Design review of the part built by this model. Coordinates are the model's own, in mm. A direction names the side the tool comes from. Give positions to 0.01 mm unless a question says otherwise; leave off trailing zeros. Write each loop counter-clockwise with the first axis right and the second up, starting at its lowest first coordinate (ties: lowest second). Pieces come first, ordered by that corner, then holes. Notation, with made-up numbers: M 39,78 L 61,78 A10 ccw 61,87 Z; hole C -28,6.25 d3. An arc over 180 degrees is marked long. Answer in a Markdown table with one row per item.
Autodesk Fusion 360 part; units mm, degrees
sketch "Sketch1" plane through (0, 0, 0) normal (0, 1, 0) x (1, 0, 0)
  line L0 (15, 32.5) -> (-15, 32.5)
  line L1 (-15, 32.5) -> (-15, -32.5)
  line L2 (-15, -32.5) -> (15, -32.5)
  line L3 (15, -32.5) -> (15, 32.5)
  line L4 (15, 32.5) -> (-15, -32.5) construction
  line L5 (-15, 32.5) -> (15, -32.5) construction
  dimension "d1" = 30
  dimension "d2" = 65
extrude "Extrude1" add sketch "Sketch1" along normal blind 2
sketch "Sketch2" plane through (0, 2, 0) normal (0, 1, 0) x (-1, 0, 0)
  line L0 (-15, 32.5) -> (-15, -32.5)
  line L1 (-15, -32.5) -> (15, -32.5)
  line L2 (15, -32.5) -> (15, 32.5)
  line L3 (15, 32.5) -> (-15, 32.5)
  circle A0 centre (-11.5, -29) radius 2.8
  circle A1 centre (11.5, -29) radius 2.8
  circle A2 centre (-11.5, 29) radius 2.8
  circle A3 centre (11.5, 29) radius 2.8
  dimension "d5" = 5.6
  dimension "d6" = 3.5
  dimension "d7" = 3.5
  dimension "d8" = 5.6
  dimension "d9" = 3.5
  dimension "d10" = 3.5
  dimension "d11" = 5.6
  dimension "d12" = 3.5
  dimension "d13" = 3.5
  dimension "d14" = 5.6
  dimension "d15" = 3.5
  dimension "d16" = 3.5
extrude "Extrude2" add sketch "Sketch2" along normal blind 21 contours A0 | A1 | A2 | A3
sketch "Sketch3" plane through (0, 23, 0) normal (0, 1, 0) x (-1, 0, 0)
  circle A0 centre (-11.5, -29) radius 2.8
  circle A1 centre (-11.5, -29) radius 1.2
  circle A2 centre (11.5, -29) radius 1.2
  circle A3 centre (11.5, -29) radius 2.8
  circle A4 centre (-11.5, 29) radius 1.2
  circle A5 centre (-11.5, 29) radius 2.8
  circle A6 centre (11.5, 29) radius 1.2
  circle A7 centre (11.5, 29) radius 2.8
  dimension "d19" = 2.4
  dimension "d20" = 2.4
  dimension "d21" = 2.4
  dimension "d22" = 2.4
extrude "Extrude3" cut sketch "Sketch3" against normal blind 5 contours A1 | A2 | A4 | A6
sketch "Sketch4" plane through (0, 2, 0) normal (0, 1, 0) x (-1, 0, 0)
  circle A0 centre (11.5, -29) radius 2.8
  circle A1 centre (11.5, 29) radius 2.8
  circle A2 centre (-11.5, -29) radius 2.8
  circle A3 centre (-11.5, 29) radius 2.8
  line L0 (-15, 32.5) -> (-15, -32.5)
  line L1 (-15, -32.5) -> (15, -32.5)
  line L2 (15, -32.5) -> (15, 32.5)
  line L3 (15, 32.5) -> (-15, 32.5)
  line L4 (-14, 26) -> (-8.4, 26)
  line L5 (-8.4, 26) -> (-8.4, -24)
  line L6 (-8.4, -24) -> (-14, -24)
  line L7 (-14, -24) -> (-14, 26)
  dimension "d25" = 5.6
  dimension "d26" = 6.5
  dimension "d27" = 1
  dimension "d28" = 50
extrude "Extrude4" cut sketch "Sketch4" against normal blind 5 contours L4 L5 L6 L7
sketch "Sketch5" plane through (0, 2, 0) normal (0, 1, 0) x (-1, 0, 0)
  line L0 (-8.4, 26) -> (-8.4, -24)
  line L1 (-8.4, -24) -> (-14, -24)
  line L2 (-14, -24) -> (-14, 26)
  line L3 (-14, 26) -> (-8.4, 26)
  circle A0 centre (11.5, -29) radius 2.8
  circle A1 centre (11.5, 29) radius 2.8
  circle A2 centre (-11.5, -29) radius 2.8
  circle A3 centre (-11.5, 29) radius 2.8
  line L4 (-15, 32.5) -> (-15, -32.5)
  line L5 (-15, -32.5) -> (15, -32.5)
  line L6 (15, -32.5) -> (15, 32.5)
  line L7 (15, 32.5) -> (-15, 32.5)
  line L8 (-14, -18) -> (-8, -18)
  line L9 (-8, -18) -> (-8, -16)
  line L10 (-8, -16) -> (-14, -16)
  line L11 (-14, -16) -> (-14, -18)
  dimension "d31" = 6
  dimension "d32" = 2
extrude "Extrude5" add sketch "Sketch5" against normal blind 2 contours L0 L2 L8 L10 L11
sketch "Sketch6" plane through (0, 2, 0) normal (0, 1, 0) x (-1, 0, 0)
  line L0 (-14, -16) -> (-14, 26)
  line L1 (-14, 26) -> (-8.4, 26)
  line L2 (-8.4, 26) -> (-8.4, -16)
  line L3 (-8.4, -16) -> (-14, -16)
  line L4 (-14, -18) -> (-8.4, -18)
  line L5 (-8.4, -18) -> (-8.4, -24)
  line L6 (-8.4, -24) -> (-14, -24)
  line L7 (-14, -24) -> (-14, -18)
  circle A0 centre (11.5, -29) radius 2.8
  circle A1 centre (11.5, 29) radius 2.8
  circle A2 centre (-11.5, -29) radius 2.8
  circle A3 centre (-11.5, 29) radius 2.8
  line L8 (-15, 32.5) -> (-15, -32.5)
  line L9 (-15, -32.5) -> (15, -32.5)
  line L10 (15, -32.5) -> (15, 32.5)
  line L11 (15, 32.5) -> (-15, 32.5)
  line L12 (10, 20) -> (-2, 20)
  line L13 (-2, 20) -> (-2, -20)
  line L14 (-2, -20) -> (10, -20)
  line L15 (10, -20) -> (10, 20)
extrude "Extrude6" cut sketch "Sketch6" against normal blind 2 contours L12 L13 L14 L15
sketch "Sketch7" plane through (0, 2, 0) normal (0, 1, 0) x (-1, 0, 0)
  line L0 (-2, 20) -> (10, 20)
  line L1 (10, 20) -> (10, -20)
  line L2 (10, -20) -> (-2, -20)
  line L3 (-2, -20) -> (-2, 20)
  line L4 (-14, -16) -> (-14, 26)
  line L5 (-14, 26) -> (-8.4, 26)
  line L6 (-8.4, 26) -> (-8.4, -16)
  line L7 (-8.4, -16) -> (-14, -16)
  line L8 (-14, -18) -> (-8.4, -18)
  line L9 (-8.4, -18) -> (-8.4, -24)
  line L10 (-8.4, -24) -> (-14, -24)
  line L11 (-14, -24) -> (-14, -18)
  circle A0 centre (11.5, -29) radius 2.8
  circle A1 centre (11.5, 29) radius 2.8
  circle A2 centre (-11.5, -29) radius 2.8
  circle A3 centre (-11.5, 29) radius 2.8
  line L12 (-15, 32.5) -> (-15, -32.5)
  line L13 (-15, -32.5) -> (15, -32.5)
  line L14 (15, -32.5) -> (15, 32.5)
  line L15 (15, 32.5) -> (-15, 32.5)
  line L16 (-8, -31) -> (4, -31)
  line L17 (4, -31) -> (4, -25)
  line L18 (4, -25) -> (-8, -25)
  line L19 (-8, -25) -> (-8, -31)
extrude "Extrude7" cut sketch "Sketch7" against normal blind 2 contours L16 L17 L18 L19
1) For faces 4 (the face through (0, 1, -32.5)), 5 (the face through (-13.01, 12.35, -31.36)), 6 (the face through (8.4, 1, -21)), list the 3-axis set-ups (+Z, -Z, +X, -X, +Y, -Y) from which the entire face can be reached by the end or side of a thin tool; tool diameter is ignored.
Geometry says:
| item | result |
|---|---|
| face 4 | -Z, +X, -X, +Y, -Y |
| face 5 | +Y |
| face 6 | +Y, -Y |
2) To check wall thickness, follow probe 1 along Z at (x, y) = (-11.5, 19.4); probe 2 along Y at (x, z) = (-11, -10.5); probe 3 along Z at (x, y) = (-14, 8.25). State the ranges of each line that lie inside material, in increasing order. Write a range as [from, to].
Geometry says:
| item | result |
|---|---|
| probe 1 | [-31.8, -30.2], [-27.8, -26.2], [26.2, 27.8], [30.2, 31.8] |
| probe 2 | [0, 2] |
| probe 3 | [-30.26, -27.74], [27.74, 30.26] |
3) Add section A-A (x = 11.5). Write out the cut boundary in (y, z).
Geometry says:
| item | result |
|---|---|
| outline | M 0,-32.5 L 2,-32.5 L 2,-31.8 L 23,-31.8 L 23,-30.2 L 18,-30.2 L 18,-27.8 L 23,-27.8 L 23,-26.2 L 2,-26.2 L 2,-24 L 0,-24 Z; M 0,-18 L 2,-18 L 2,-16 L 0,-16 Z; M 0,26 L 2,26 L 2,26.2 L 23,26.2 L 23,27.8 L 18,27.8 L 18,30.2 L 23,30.2 L 23,31.8 L 2,31.8 L 2,32.5 L 0,32.5 Z |
4) The part is to be moulded in two halves that separate along X. For faces 1 (the face through (3, 0, 0)), 2 (the face through (-11, 18, 29)), 3 (the face through (-12.645, 20.535, 29.36)), say which applies: released by +X, released by -X, zero draft, split by the parting line, or undercut.
Geometry says:
| item | result |
|---|---|
| face 1 | zero draft |
| face 2 | undercut |
| face 3 | undercut |
5) Insertion check: P1, Ø0.7, axis at x = 12, z = 29, coming from the +Y side; P2, Ø3, axis at x = -10.5, z = 17, coming from the +Y side; P3, Ø1.5, axis at x = 2, z = 17, coming from the -Y side. Each pin has a flat end and moves straight along its axis. Give the tip position at first contact, or say it passes through.
Geometry says:
| item | result |
|---|---|
| P1 | y = 18 |
| P2 | y = 2 |
| P3 | y = 0 |
6) Add section D-D (z = 11). Write out the cut boundary in (x, y), and give its area (3 significant figures).
Geometry says:
| item | result |
|---|---|
| outline | M -15,0 L -10,0 L -10,2 L -15,2 Z; M 2,0 L 8.4,0 L 8.4,2 L 2,2 Z; M 14,0 L 15,0 L 15,2 L 14,2 Z |
| area | 24.8 mm^2 |
7) Add section B-B (z = -29). Write out the cut boundary in (x, y), and give its area (3 significant figures).
Geometry says:
| item | result |
|---|---|
| outline | M -15,0 L -4,0 L -4,2 L -8.7,2 L -8.7,23 L -10.3,23 L -10.3,18 L -12.7,18 L -12.7,23 L -14.3,23 L -14.3,2 L -15,2 Z; M 8,0 L 15,0 L 15,2 L 14.3,2 L 14.3,23 L 12.7,23 L 12.7,18 L 10.3,18 L 10.3,23 L 8.7,23 L 8.7,2 L 8,2 Z |
| area | 247 mm^2 |
8) Add section C-C (x = -5.75). Write out the cut boundary in (y, z), and give its area (3 significant figures).
Geometry says:
| item | result |
|---|---|
| outline | M 0,-32.5 L 2,-32.5 L 2,-20 L 0,-20 Z; M 0,20 L 2,20 L 2,32.5 L 0,32.5 Z |
| area | 50.0 mm^2 |
